For this review, take the finished solid that the model builds, in its own axes (mm). Face numbers are marked on the shaded views. A direction names the side the tool comes from. Give positions to 0.01 mm unless a question says otherwise; leave off trailing zeros. Loops run counter-clockwise (first coordinate to the right, second up) from the corner with the lowest first, then second, coordinate; pieces in that order, holes last. Notation, with made-up numbers: (3, -16.75) - (61, -16.75) arc R12 ccw to (61, -1.75) - close; hole circle Ø9 at (57.25, -16.5). An arc over 180 degrees is marked (long way). Put each result on its own line as item: value. Start each with the question number.
from build123d import *

# Parameters (mm, degrees)
F0_R     = 3.81
F1_DEPTH = 25.4
F2_R     = 6.35
F2_R_2   = 3.81
F3_DEPTH = 3.81
F2_R_3   = 12.7
F4_DEPTH = 3.81


# Not quite as in the source:
# - a fillet or chamfer that OpenCascade refuses, or shapes differently, is made with other operations: its cross-section is extruded or revolved along the edge and cut away or added


with BuildPart() as f1:
    # F0 (on Top) → F1 (new body)
    with BuildSketch(Plane.XY):
        Circle(F0_R)
    extrude(amount=F1_DEPTH)

    # F2 (on face) → F3 (join)
    with BuildSketch(Plane.XY.offset(25.4)):
        Circle(F2_R)
        Circle(F2_R_2, mode=Mode.SUBTRACT)
        Circle(F2_R_2)
    extrude(amount=F3_DEPTH)

    # F2 (on face) → F4 (join)
    with BuildSketch(Plane.XY.offset(25.4)):
        Circle(F2_R_3)
        Circle(F2_R, mode=Mode.SUBTRACT)
    extrude(amount=F4_DEPTH)

    # F5: fillet of radius 5.08 on 1 edges, made by hand

    # F5_s1 → F5_t2 (revolve, cut)
    with BuildSketch(Plane.XZ):
        with BuildLine():
            ThreePointArc((12.7, 25.4), (10.8921631237, 28.1460926284), (7.7813111503, 29.21))
            Line((7.7813111503, 29.21), (12.7, 29.21))
            Line((12.7, 29.21), (12.7, 25.4))
        make_face()
    revolve(axis=Axis((0, 0, 29.21), (0, 0, 1)), mode=Mode.SUBTRACT)


solid = f1.part
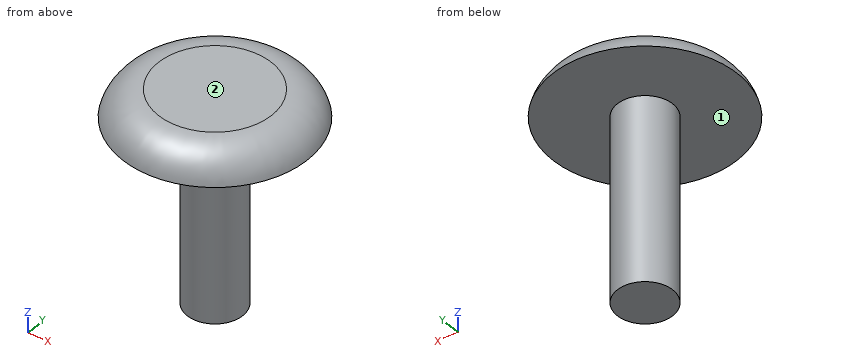
1) Take a section at C-C on z = 25. State the section outline as (x, y) points.
2) Machinability: for the marked faces 1 and 2, which of the approach directions +Z, -Z, +X, -X, +Y, -Y give a long, thin tool a straight path to every point of the face, cutting with its end or side? Answer none if there is none.
3) Wall thickness on probe 1 along Z at (x, y) = (9.75, 4.75); probe 2 along X at (y, z) = (3, 24); probe 3 along Z at (x, y) = (-9.5, 6.75): over which ranges is each line inside the solid? List them lowest first.
4) Insertion check: P1, Ø1, axis at x = -2, y = -5.5, coming from the -Z side; P2, Ø5, axis at y = 4.5, z = 18.5, coming from the -X side; P3, Ø12, axis at x = -1.5, z = 18.5, coming from the -Y side. Each pin has a flat end and moves straight along its axis. Give the tip position at first contact, or say it passes through.
5) Take a section at A-A on y = 0. State the section outline as (x, z) points, and give its area (3 significant figures).
Answers follow:
1. outline: circle Ø7.62 at (0, 0)
2. face 1: -Z
2. face 2: +Z, +X, -X, +Y, -Y
3. probe 1: 25.4 to 28.18
3. probe 2: -2.35 to 2.35
3. probe 3: 25.4 to 27.42
4. P1: z = 25.4
4. P2: x = -3.24
4. P3: y = -3.81
5. outline: (-12.7, 25.4) - (-3.81, 25.4) - (-3.81, 0) - (3.81, 0) - (3.81, 25.4) - (12.7, 25.4) arc R5.08 ccw to (7.78, 29.21) - (-7.78, 29.21) arc R5.08 ccw to start
5. area: 281 mm2
